Could you check a few things on this model? Use its own coordinates, in mm. A direction names the side the tool comes from. Coordinates: 2 decimals unless noted, no trailing zeros. Loops run counter-clockwise (first coordinate to the right, second up) from the corner with the lowest first, then second, coordinate; pieces in that order, holes last.
from build123d import *

# Parameters (mm, degrees)
SKETCH1_W           = 28.575
SKETCH1_H           = 19.05
BOSS_EXTRUDE1_DEPTH = 12.7
SKETCH2_R           = 3.175
BOSS_EXTRUDE2_DEPTH = 17.4625
SKETCH3_R           = 1.905
CUT_EXTRUDE1_DEPTH  = 49.645932191


with BuildPart() as part:
    # Sketch1 → Boss-Extrude1 (new, symmetric)
    with BuildSketch(Plane(origin=(0, 0, 0), x_dir=(1, 0, 0), z_dir=(0, 1, 0))):
        with Locations((-14.2875, 0)):
            Rectangle(SKETCH1_W, SKETCH1_H)
        Polygon((0, 9.525), (0, -9.525), (0, -11.1125), (36.5125, -11.1125), (36.5125, 11.1125), (0, 11.1125), align=None)
    extrude(amount=BOSS_EXTRUDE1_DEPTH, both=True)

    # Sketch2 → Boss-Extrude2 (add, symmetric)
    with BuildSketch(Plane.XZ):
        with Locations(Location((25.4, 0, 0), (0, 0, 90))):
            Circle(SKETCH2_R)
    extrude(amount=BOSS_EXTRUDE2_DEPTH, both=True)

    # Sketch3 → Cut-Extrude1 (cut, through all)
    with BuildSketch(Plane.XZ.offset(12.7)):
        with Locations(Location((5.55625, 7.9375, 0), (0, 0, 270))):
            Circle(SKETCH3_R)
        with Locations(Location((5.55625, -7.9375, 0), (0, 0, 270))):
            Circle(SKETCH3_R)
    extrude(amount=-CUT_EXTRUDE1_DEPTH, mode=Mode.SUBTRACT)


solid = part.part
(1) Imagine slicing it at A-A, the plane x = 25.4. Write out the boundary of the cut face in (y, z) (1 decimal).
Answers:
outline: (-17.5, -3.2) - (-12.7, -3.2) - (-12.7, -11.1) - (12.7, -11.1) - (12.7, -3.2) - (17.5, -3.2) - (17.5, 3.2) - (12.7, 3.2) - (12.7, 11.1) - (-12.7, 11.1) - (-12.7, 3.2) - (-17.5, 3.2) - close
(2) Imagine slicing it at D-D, the plane z = 0. Write out the boundary of the cut face in (x, y) (1 decimal).
Answers:
outline: (-28.6, -12.7) - (22.2, -12.7) - (22.2, -17.5) - (28.6, -17.5) - (28.6, -12.7) - (36.5, -12.7) - (36.5, 12.7) - (28.6, 12.7) - (28.6, 17.5) - (22.2, 17.5) - (22.2, 12.7) - (-28.6, 12.7) - close
(3) I need wall thicknesses on probe 1 along Z at (x, y) = (6.5, 6); probe 2 along Y at (x, z) = (31, 3.25); probe 3 along X at (y, z) = (11.5, -10). Which ranges of each line are inside material? Lowest first, please.
Answers:
probe 1: z = -11.11 to -9.59, -6.28 to 6.28, 9.59 to 11.11
probe 2: y = -12.7 to 12.7
probe 3: x = 0 to 36.51
(4) For pin 1 (12.5 mm diameter, centred on x = -14, y = -1.5, fed in from +Z) (3 decimals); pin 2 (1.7 mm diameter, centred on y = 0.5, z = 10.5, fed in from -X); pin 3 (4 mm diameter, centred on x = 2.5, z = 5, fed in from -Y), each with a flat end and sliding along its axis, tell me the tip position at first contact or that it passes through.
Answers:
pin 1: stops at z = 9.525
pin 2: stops at x = 0
pin 3: stops at y = -12.7
(5) We'd pull the mould along Z, two halves only. Please class faces 1 (the face through (0, 0, -10)), 2 (the face through (18, 0, 11.112)), 3 (the face through (3.87, -0.18, -8.82)): +Z half, -Z half, draft (parallel to the pull), parting line (faces both ways), or undercut.
Answers:
face 1: draft
face 2: +Z half
face 3: undercut
(6) Imagine slicing it at B-B, the plane y = -0.5. Write out the boundary of the cut face in (x, z) (1 decimal).
Answers:
outline: (-28.6, -9.5) - (0, -9.5) - (0, -11.1) - (36.5, -11.1) - (36.5, 11.1) - (0, 11.1) - (0, 9.5) - (-28.6, 9.5) - close; hole circle Ø3.8 at (5.6, -7.9); hole circle Ø3.8 at (5.6, 7.9)
(7) Imagine slicing it at C-C, the plane z = 8. Write out the boundary of the cut face in (x, y) (1 decimal).
Answers:
outline: (-28.6, -12.7) - (3.7, -12.7) - (3.7, 12.7) - (-28.6, 12.7) - close; (7.5, -12.7) - (36.5, -12.7) - (36.5, 12.7) - (7.5, 12.7) - close
(8) Which directions (+Z, -Z, +X, -X, +Y, -Y) give clear straight access to the entire face, cutting with the end or side of a thin tool? Please do faces 4 (the face through (22.25, -15.11, -0.41)), 5 (the face through (-14, 0, 9.525)), 6 (the face through (22.25, 15.05, -0.41)).
Answers:
face 4: -Y
face 5: +Z, -X, +Y, -Y
face 6: +Y
